For this review, use the dimensioned drawing (mm, ordinates from the lowest corner) and the shaded views. Give positions to 0.01 mm unless a question says otherwise; leave off trailing zeros. Order: outer loops, then holes, each group sorted by start corner. A loop starts at its lowest first (then second) coordinate and runs counter-clockwise, first axis right, second up. Notation, with made-up numbers: M 82.5,18.25 L 113.5,18.25 A20 cw 113.5,36.25 Z; hole C 69.5,-22 d2. An arc over 180 degrees is marked long. One line per question, with ' | ' between items. Start each with the question number.
1. Wall thickness on L1, parallel to Y at x = 25, z = 3.75; L2, parallel to Y at x = 52, z = 7.25; L3, parallel to Y at x = 29, z = 6: over which ranges is each line inside the solid? List them lowest first.
2. Insertion check: P1, Ø10, axis at x = 25, y = 25, coming from the -Z side. The pin has a flat end and moves straight along its axis. Give the tip position at first contact, or say it passes through.
3. We need section C-C on z = 5.25. Write out the cut boundary in (x, y), then the cut area to 3 significant figures.
4. We need section A-A on x = 25. Write out the cut boundary in (y, z).
5. We need section B-B on y = 25. Write out the cut boundary in (x, z), then the cut area to 3 significant figures.
6. We need section D-D on x = 6. Write out the cut boundary in (y, z).
7. The part is to be moulded in two halves that separate along Y. For the marked faces 1, 2 and 3, say which applies: +Y half, -Y half, draft (parallel to the pull), parting line (faces both ways), or undercut.
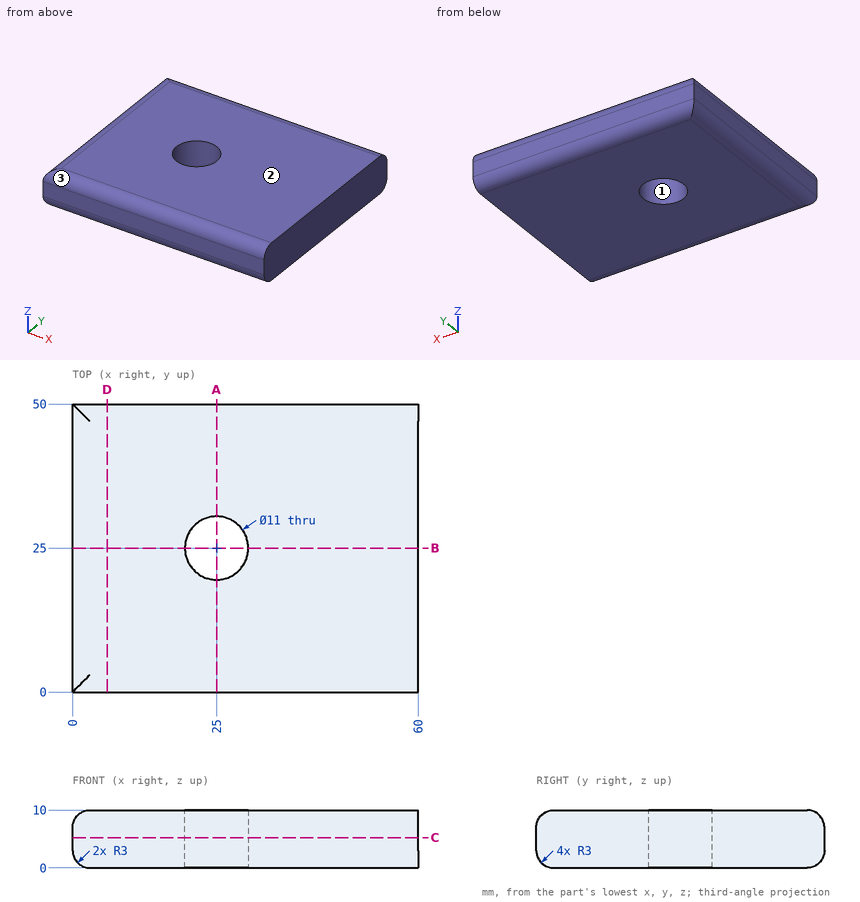
Entries:
1) L1: y = 0 to 19.5, 30.5 to 50 | L2: y = 0.01 to 49.99 | L3: y = 0 to 21.23, 28.77 to 50
2) P1: passes through
3) outline: M 0,0 L 60,0 L 60,50 L 0,50 Z; hole C 25,25 d11 | area: 2,900 mm^2
4) outline: M 0,3 A3 ccw 3,0 L 19.5,0 L 19.5,10 L 3,10 A3 ccw 0,7 Z; M 30.5,0 L 47,0 A3 ccw 50,3 L 50,7 A3 ccw 47,10 L 30.5,10 Z
5) outline: M 0,3 A3 ccw 3,0 L 19.5,0 L 19.5,10 L 3,10 A3 ccw 0,7 Z; M 30.5,0 L 60,0 L 60,10 L 30.5,10 Z | area: 486 mm^2
6) outline: M 0,3 A3 ccw 3,0 L 47,0 A3 ccw 50,3 L 50,7 A3 ccw 47,10 L 3,10 A3 ccw 0,7 Z
7) face 1: undercut | face 2: draft | face 3: -Y half
